Check sheet for the modelled part. Datum: model origin and axes. Units: mm. A direction names the side the tool comes from. Coordinates: 2 decimals unless noted, no trailing zeros. Order: outer loops, then holes, each group sorted by start corner. A loop starts at its lowest first (then second) coordinate and runs counter-clockwise, first axis right, second up. Notation, with made-up numbers: (88, 70.25) -> (112, 70.25) arc R10 ccw to (112, 81.25) -> close; hole circle Ø4 at (89, 7.5). An arc over 180 degrees is marked (long way). Put each result on its own line as item: value. Start each with the question number.
```python
from build123d import *

# Parameters (mm, degrees)
F1_DEPTH  = 112.7125
F2_T      = -1.524
F5_DEPTH  = 225.425
F7_DEPTH  = 225.425
F8_R      = 51.8099901909
F9_DEPTH  = 225.425
F14_W     = 1.27
F14_H     = 1.8664713708
F15_DEPTH = 225.425
F16_R     = 0.508
F17_R     = 6.35
F18_R     = 0.254


with BuildPart() as f1:
    # F0 (on Right) → F1 (new body, symmetric)
    with BuildSketch(Plane.YZ):
        with BuildLine():
            Line((-72.136, 14.4276117903), (-26.3105725372, -25.4078245579))
            Line((-26.3105725372, -25.4078245579), (0, 0))
            Line((0, 0), (0, 37.338))
            ThreePointArc((0, 37.338), (-36.8647965725, 36.3151722047), (-68.7392263709, 17.7657752319))
            Line((-68.7392263709, 17.7657752319), (-72.136, 14.4276117903))
        make_face()
    extrude(amount=F1_DEPTH, both=True)

    # F2
    f2_openings = [f1.faces().sort_by_distance(p)[0] for p in [
        (0, -49.223286, -5.490106),
        (-112.7125, -29.609995, 11.681685),
        (112.7125, -29.609995, 11.681685),
    ]]
    offset(amount=F2_T, openings=f2_openings)

    # F4 (on face) → F5 (join, through all)
    with BuildSketch(Plane(origin=(-112.7125, 0, 0), x_dir=(0, -1, 0), z_dir=(-1, 0, 0))):
        Polygon((69.0653059094, 11.7582981414), (70.9822682431, 13.424688075), (69.170655641, 15.2050419106), (67.2536933072, 13.5386519769), align=None)
    extrude(amount=-F5_DEPTH)

    # F6 (on face) → F7 (join, through all)
    with BuildSketch(Plane(origin=(-112.7125, 0, 0), x_dir=(0, -1, 0), z_dir=(-1, 0, 0))):
        Polygon((27.5549826692, -20.9733491998), (25.6380203354, -22.6397391335), (27.4651434283, -24.4041713944), (29.382105762, -22.7377814608), align=None)
    extrude(amount=-F7_DEPTH)

    # F8 (on face) → F9 (cut, through all)
    with BuildSketch(Plane(origin=(-112.7125, 0, 0), x_dir=(0, -1, 0), z_dir=(-1, 0, 0))):
        with Locations((76.7665722185, -37.1750323717)):
            Circle(F8_R)
    extrude(amount=-F9_DEPTH, mode=Mode.SUBTRACT)

    # F10 (on face) + F11 (on face) + F12 (on face) + F13 (on face) + F14 (on face) → F15 (join, through all)
    with BuildSketch(Plane(origin=(-112.7125, 0, 0), x_dir=(0, -1, 0), z_dir=(-1, 0, 0))):
        Polygon((23.17140416, -20.2577555812), (24.0849657065, -21.1399717116), (25.5666650167, -19.8519501518), (24.530017001, -18.8508707997), align=None)
    with BuildSketch(Plane(origin=(-112.7125, 0, 0), x_dir=(0, -1, 0), z_dir=(-1, 0, 0))):
        Polygon((23.6164554546, -17.9686546692), (25.5666650167, -19.8519501518), (26.4488811472, -18.9383886054), (24.498671585, -17.0550931227), align=None)
    with BuildSketch(Plane(origin=(-112.7125, 0, 0), x_dir=(0, -1, 0), z_dir=(-1, 0, 0))):
        Polygon((65.7138225954, 15.0519527371), (67.6307849291, 16.7183426707), (66.724978628, 17.6085195885), (64.8080162943, 15.9421296549), align=None)
    with BuildSketch(Plane(origin=(-112.7125, 0, 0), x_dir=(0, -1, 0), z_dir=(-1, 0, 0))):
        Polygon((13.0308709947, -10.4651565328), (13.9444325411, -11.3473726633), (15.303045382, -9.9404878818), (16.2166069285, -10.8227040123), (17.098823059, -9.9091424658), (15.2716999661, -8.1447102049), align=None)
    with BuildSketch(Plane(origin=(-112.7125, 0, 0), x_dir=(0, -1, 0), z_dir=(-1, 0, 0))):
        Polygon((1.524, 23.2821790422), (1.524, 22.0121790422), (4.7498, 22.0121790422), (4.7498, 24.5521790422), (3.4798, 24.5521790422), (3.4798, 23.2821790422), align=None)
        with Locations((4.1148, 35.7724147276)):
            Rectangle(F14_W, F14_H)
    extrude(amount=-F15_DEPTH)

    # F16
    f16_edges = [f1.edges().sort_by_distance(p)[0] for p in [
        (0, -26.310573, -25.407825),
        (0, -72.136, 14.427612),
        (0, 0, 37.338),
    ]]
    fillet(f16_edges, radius=F16_R)

    # F17
    f17_edges = [f1.edges().sort_by_distance(p)[0] for p in [
        (0, -1.524, 0.6469),
        (0, 0, 0),
    ]]
    fillet(f17_edges, radius=F17_R)

    # F18
    f18_edges = [f1.edges().sort_by_distance(p)[0] for p in [
        (0, -27.554983, -20.973349),
        (0, -67.567953, 13.811833),
    ]]
    fillet(f18_edges, radius=F18_R)


solid = f1.part
```
1) Access from +Z, -Z, +X, -X, +Y, -Y to the whole of each face (thin tool, end or side, straight path). Record for faces 4 (the cylindrical face through (1.578, -37.517, 34.536)), 5 (the cylindrical face through (1.578, -2.015, 0.894)), 6 (the cylindrical face through (1.58, -36.56, 36.4)).
2) Sectioned sample at B-B (y = -47). Record the boundary of the cut face in (x, z).
3) Sectioned sample at C-C (z = 5.5). Record the boundary of the cut face in (x, y).
4) Mould release check, pull along Z, two halves, no side actions. Record for faces 1 (the flat face through (112.712, -4, 24)), 2 (the flat face through (2, -1.524, 13)), 3 (the cylindrical face through (1.58, -0.49, 0.25)): +Z half, -Z half, draft (parallel to the pull), parting line (faces both ways), or undercut.
5) Scan lines: line 1 along Y through (x, z) = (102.5, 21.5); line 2 along Z through (x, y) = (-3.5, -5); line 3 along Y through (x, z) = (72, 4). Record each from-to range of solid material in increasing order. Write a range as [from, to].
6) Gauge pin test, flat ends, axial feed: pin 1 (2 mm diameter, centred on x = 25.5, z = 23.5, fed in from -Y); pin 2 (5 mm diameter, centred on x = -41, y = -33.5, fed in from -Z); pin 3 (1 mm diameter, centred on x = -50.5, y = -3, fed in from +Z). Record the tip position at first contact, or that the pin passes through.
Entries:
1. face 4: +X, -X
1. face 5: +X, -X, -Y
1. face 6: +Z, +X, -X
2. outline: (-112.71, 30.94) -> (112.71, 30.94) -> (112.71, 32.62) -> (-112.71, 32.62) -> close
3. outline: (-112.71, -1.52) -> (112.71, -1.52) -> (112.71, 0) -> (-112.71, 0) -> close
4. face 1: draft
4. face 2: undercut
4. face 3: -Z half
5. line 1: y = [-64.65, -62.25], [-1.52, 0]
5. line 2: z = [-4.83, -2.71], [36.75, 38.29]
5. line 3: y = [-1.52, 0]
6. pin 1: stops at y = -63.44
6. pin 2: stops at z = 34.98
6. pin 3: stops at z = 38.04
